Autodesk Inventor part; units mm, degrees
ref_plane "YZ Plane" through (0, 0, 0) normal (1, 0, 0) x (0, 1, 0)
ref_plane "XZ Plane" through (0, 0, 0) normal (0, 1, 0) x (-1, 0, 0)
ref_plane "XY Plane" through (0, 0, 0) normal (0, 0, 1) x (1, 0, 0)
sketch "Sketch1" plane through (0, 0, 0) normal (0, 0, 1) x (1, 0, 0)
  line L0 (-10, -0.3003) -> (50, -0.3003)
  line L1 (50, -0.3003) -> (50, -60.3003)
  line L2 (50, -60.3003) -> (-10, -60.3003)
  line L3 (-10, -60.3003) -> (-10, -0.3003)
  line L4 (-11.6, 1.2997) -> (51.6, 1.2997)
  line L5 (51.6, 1.2997) -> (51.6, -61.9003)
  line L6 (51.6, -61.9003) -> (-11.6, -61.9003)
  line L7 (-11.6, -61.9003) -> (-11.6, 1.2997)
  point P0 (-10, -30.3003)
  point P1 (-11.6, -30.3003)
  dimension "d1" = 60
  dimension "d2" = 60
  dimension "d3" = 1.6
  dimension "d4" = 1.6
  dimension "d5" = 1.6
  dimension "d6" = 1.6
extrude "Extrusion1" add sketch "Sketch1" along normal blind 20 contours L0 L1 L2 L3 | L4 L5 L6 L7
sketch "Sketch2" plane through (0, 0, 0) normal (0, 0, -1) x (-1, 0, 0)
  line L0 (-50, -0.3003) -> (10, -0.3003)
  line L1 (10, -0.3003) -> (10, -60.3003)
  line L2 (10, -60.3003) -> (-50, -60.3003)
  line L3 (-50, -60.3003) -> (-50, -0.3003)
  line L4 (-51.6, 1.2997) -> (11.6, 1.2997)
  line L5 (11.6, -61.9003) -> (-51.6, -61.9003)
  line L6 (-51.6, -61.9003) -> (-51.6, 1.2997)
  line L7 (11.6, 1.2997) -> (11.6, -61.9003)
  point P0 (0, 0)
  dimension "d9" = 60
  dimension "d10" = 1.6
  dimension "d11" = 1.6
  dimension "d12" = 1.6
  dimension "d61" = 1.6
extrude "Extrusion2" cut sketch "Sketch2" against normal blind 18.4 contours L0 L1 L2 L3
sketch "Sketch3" plane through (-11.6, -61.9003, 0) normal (0, -1, 0) x (1, 0, 0)
  line L0 (57.6038, 13.4) -> (47.6038, 13.4)
  line L1 (47.6038, 13.4) -> (47.6038, 18.4)
  line L2 (47.6038, 18.4) -> (57.6038, 18.4)
  line L3 (57.6038, 18.4) -> (57.6038, 13.4)
  line L4 (0, 20) -> (63.2, 20)
  point P0 (11.6, 0)
  point P1 (52.6038, 18.4)
  dimension "d15" = 10
  dimension "d16" = 5
  dimension "d17" = 1.6
extrude "Extrusion3" cut sketch "Sketch3" against normal blind 18.4
fillet "Fillet1" radius 2 1 edges at (-11.6, -61.9003, 10)
fillet "Fillet2" radius 2 3 edges at (-11.6, 1.2997, 10) (51.6, 1.2997, 10) (51.6, -61.9003, 10)
fillet "Fillet3" radius 2 8 edges at (51.0142, -61.3145, 20) (51.6, -30.3003, 20) (51.0142, 0.7139, 20) (20, 1.2997, 20) (-11.0142, 0.7139, 20) (-11.6, -30.3003, 20) (-11.0142, -61.3145, 20) (20, -61.9003, 20)
sketch "Sketch4" plane through (-11.6, -59.9003, 0) normal (-1, 0, 0) x (0, 0, 1)
  line L0 (14.4, 37.5852) -> (18.4, 37.5852)
  line L1 (18.4, 37.5852) -> (18.4, 45.5852)
  line L2 (18.4, 45.5852) -> (14.4, 45.5852)
  line L3 (14.4, 45.5852) -> (14.4, 37.5852)
  line L4 (20, 0) -> (20, 59.2)
  point P0 (0, 59.9003)
  point P1 (18.4, 41.5852)
  dimension "d23" = 4
  dimension "d24" = 8
  dimension "d25" = 1.6
extrude "Extrusion4" cut sketch "Sketch4" against normal blind 18.4
sketch "Sketch5" plane through (0, 0, 18.4) normal (0, 0, -1) x (-1, 0, 0)
  point P0 (0, 0)
sketch "Sketch6" plane through (0, 0, 18.4) normal (0, 0, -1) x (-1, 0, 0)
  point P0 (0, 0)
fillet "Fillet4" radius 2 4 edges at (50, -0.3003, 9.2) (-10, -0.3003, 9.2) (-10, -60.3003, 9.2) (50, -60.3003, 9.2)
sketch "Sketch7" plane through (0, 0, 18.4) normal (0, 0, -1) x (-1, 0, 0)
  point P0 (0, 0)
sketch "Sketch8" plane through (0, 0, 18.4) normal (0, 0, -1) x (-1, 0, 0)
  circle A0 centre (-46.25, -4.0503) radius 2.6
  circle A1 centre (6.25, -56.5503) radius 2.6
  line L0 (-48, -0.3003) -> (8, -0.3003)
  line L1 (-50, -58.3003) -> (-50, -2.3003)
  line L2 (10, -2.3003) -> (10, -58.3003)
  line L3 (8, -60.3003) -> (-48, -60.3003)
  point P0 (0, 0)
  dimension "d30" = 5.2
  dimension "d31" = 5.2
  dimension "d32" = 3.75
  dimension "d33" = 3.75
  dimension "d34" = 3.75
  dimension "d35" = 3.75
extrude "Extrusion5" add sketch "Sketch8" along normal up to surface (18.4 mm away)
sketch "Sketch9" plane through (46.25, -4.0503, 0) normal (0, 0, -1) x (-1, 0, 0)
  circle A0 centre (0, 0) radius 2.6
  point P0 (46.25, 4.0503)
hole "Hole1" at (46.25, -4.0503, 0) direction (0, 0, 1) diameter 3.8 depth 6 tip angle 118
sketch "Sketch10" plane through (-6.25, -56.5503, 0) normal (0, 0, -1) x (-1, 0, 0)
  circle A0 centre (0, 0) radius 2.6
  point P0 (-6.25, 56.5503)
hole "Hole2" at (-6.25, -56.5503, 0) direction (0, 0, 1) diameter 3.8 depth 6 tip angle 118
sketch "Sketch11" plane through (0, 0, 18.4) normal (0, 0, -1) x (-1, 0, 0)
  circle A0 centre (-9.4611, -3.3127) radius 1.25
  circle A1 centre (-9.4611, -18.5527) radius 1.25
  circle A2 centre (-31.0511, -3.3127) radius 1.25
  circle A3 centre (-31.0511, -18.5527) radius 1.25
  line L0 (-50, -58.3003) -> (-50, -2.3003)
  point P0 (0, 0)
  dimension "d54" = 2.5
  dimension "d55" = 2.5
  dimension "d56" = 2.5
  dimension "d57" = 2.5
extrude "Extrusion6" add sketch "Sketch11" along normal blind 8
properties part number "LimB_module" material "Brass"
Here's how the part is built. I have some questions about the finished solid (model axes, mm). A direction names the side the tool comes from. Give positions to 0.01 mm unless a question says otherwise; leave off trailing zeros. Order: outer loops, then holes, each group sorted by start corner. A loop starts at its lowest first (then second) coordinate and runs counter-clockwise, first axis right, second up. Notation, with made-up numbers: M 17.25,-35 L 70.25,-35 A9 ccw 70.25,-23 Z; hole C -24,27.25 d5. An arc over 180 degrees is marked long. Use a Markdown table: item, result. Add a question column.
1. If we mould it in two halves opening along X, with no side actions, what happens to faces 3 (the cylindrical face through (-11, 0.73, 9.13)), 4 (the flat face through (-11, -22.315, 16)), 5 (the cylindrical face through (-5.69, -54.01, 9.33))? For each: +X half, -X half, draft (parallel to the pull), parting line (faces both ways), or undercut.
2. Suppose I cut it at C-C (y = -38). List the corners of the cut face in (x, z) for me.
3. I need wall thicknesses on probe 1 along Y at (x, z) = (-6, 3); probe 2 along Y at (x, z) = (-6.25, 3); probe 3 along X at (y, z) = (-4, 9.25). Which ranges of each line are inside material? Lowest first, please. Write a range as from..to.
4. For pin 1 Ø0.7 at (x, y) = (9, -3) entering from -Z; pin 2 Ø0.8 at (x, z) = (-11, 17.5) entering from -Y; pin 3 Ø8 at (x, y) = (17, -33.5) entering from -Z; pin 4 Ø5 at (x, y) = (-6.25, -56.55) entering from -Z, each with a flat end and sliding along its axis, tell me the tip position at first contact or that it passes through.
5. Suppose I cut it at D-D (x = 23). List the corners of the cut face in (y, z) for me, and give its area (3 significant figures).
6. Suppose I cut it at B-B (z = 2.25). List the corners of the cut face in (x, y) for me.
7. Suppose I cut it at A-A (z = 9.5). List the corners of the cut face in (x, y) for me.
8. On a 3-axis mill with a long thin cutter (end or side, diameter ignored), from which of +Z, -Z, +X, -X, +Y, -Y can I reach the whole of each face in a straight line? I mean faces 1 (the flat face through (50, -31, 9)), 2 (the flat face through (18, -61, 0)). Say none if no direction works.
Results list:
| question | item | result |
|---|---|---|
| 1 | face 3 | -X half |
| 1 | face 4 | draft |
| 1 | face 5 | undercut |
| 2 | outline | M -11.6,0 L -10,0 L -10,18.4 L 50,18.4 L 50,0 L 51.6,0 L 51.6,18 A2 ccw 49.6,20 L -9.6,20 A2 ccw -11.6,18 Z |
| 3 | probe 1 | y = -61.9..-60.3, -59.14..-58.43, -54.67..-53.96, -0.3..1.3 |
| 3 | probe 2 | y = -61.9..-60.3, -59.15..-58.45, -54.65..-53.95, -0.3..1.3 |
| 3 | probe 3 | x = -11.6..-10, 43.65..48.85, 50..51.6 |
| 4 | pin 1 | stops at z = 10.4 |
| 4 | pin 2 | stops at y = -61.63 |
| 4 | pin 3 | stops at z = 18.4 |
| 4 | pin 4 | stops at z = 0 |
| 5 | outline | M -61.9,0 L -60.3,0 L -60.3,18.4 L -0.3,18.4 L -0.3,0 L 1.3,0 L 1.3,18 A2 ccw -0.7,20 L -59.9,20 A2 ccw -61.9,18 Z |
| 5 | area | 158 mm² |
| 6 | outline | M -11.6,-59.9 A2 ccw -9.6,-61.9 L 49.6,-61.9 A2 ccw 51.6,-59.9 L 51.6,-0.7 A2 ccw 49.6,1.3 L -9.6,1.3 A2 ccw -11.6,-0.7 Z; C -6.25,-56.55 d5.2; C 46.25,-4.05 d5.2; hole M -10,-58.3 A2 ccw -8,-60.3 L 48,-60.3 A2 ccw 50,-58.3 L 50,-2.3 A2 ccw 48,-0.3 L -8,-0.3 A2 ccw -10,-2.3 Z; hole C -6.25,-56.55 d3.8; hole C 46.25,-4.05 d3.8 |
| 7 | outline | M -11.6,-59.9 A2 ccw -9.6,-61.9 L 49.6,-61.9 A2 ccw 51.6,-59.9 L 51.6,-0.7 A2 ccw 49.6,1.3 L -9.6,1.3 A2 ccw -11.6,-0.7 Z; C -6.25,-56.55 d5.2; C 46.25,-4.05 d5.2; hole M -10,-58.3 A2 ccw -8,-60.3 L 48,-60.3 A2 ccw 50,-58.3 L 50,-2.3 A2 ccw 48,-0.3 L -8,-0.3 A2 ccw -10,-2.3 Z |
| 8 | face 1 | -Z |
| 8 | face 2 | -Z, +X, -X, +Y, -Y |
